Here's how the part is built. I have some questions about the finished solid (model axes, mm). Round coordinates to 2 decimals unless told otherwise and drop trailing zeros. Order: outer loops, then holes, each group sorted by start corner. A loop starts at its lowest first (then second) coordinate and runs counter-clockwise, first axis right, second up.
```python
from build123d import *

# Parameters (mm, degrees)
F0_R     = 31.75
F0_R_2   = 24.638
F1_DEPTH = 12.7
F2_R     = 3.175
F3_W     = 32.752518
F3_H     = 69.030817
F4_DEPTH = 15.875


with BuildPart() as f1:
    # F0 (on Front) → F1 (new body, symmetric)
    with BuildSketch(Plane.XZ):
        Circle(F0_R)
        Circle(F0_R_2, mode=Mode.SUBTRACT)
    extrude(amount=F1_DEPTH, both=True)

    # F2
    f2_edges = [f1.edges().sort_by_distance(p)[0] for p in [
        (-31.75, -12.7, 0),
        (-31.75, 12.7, 0),
    ]]
    fillet(f2_edges, radius=F2_R)

    # F3 (on Front) → F4 (cut, symmetric)
    with BuildSketch(Plane.XZ):
        with Locations((-16.376259, -0.200259)):
            Rectangle(F3_W, F3_H)
    extrude(amount=F4_DEPTH, both=True, mode=Mode.SUBTRACT)


solid = f1.part
```
1. If we mould it in two halves opening along Z, with no side actions, what happens to faces 1 (the cylindrical face through (24.632, 0.178, -0.542)), 2 (the cylindrical face through (31.742, -0.133, -0.698)), 3 (the flat face through (0, 0, 28))? For each: released by +Z, released by -Z, zero draft, split by the parting line, or undercut.
Evaluation:
face 1: undercut
face 2: split by the parting line
face 3: zero draft
2. I need wall thicknesses on probe 1 along Z at (x, y) = (16, 6); probe 2 along Z at (x, y) = (6.5, 7.5); probe 3 along X at (y, z) = (-11.5, 10). Which ranges of each line are inside material? Lowest first, please.
Evaluation:
probe 1: z = -27.42 to -18.74, 18.74 to 27.42
probe 2: z = -31.08 to -23.77, 23.77 to 31.08
probe 3: x = 22.52 to 29.41
3. If we section it at A-A, the plane z = 0: Write out the boundary of the cut face in (x, y) (3 decimals), and give its area (3 significant figures).
Evaluation:
outline: (24.638, -12.7) - (28.575, -12.7) arc R3.175 ccw to (31.75, -9.525) - (31.75, 9.525) arc R3.175 ccw to (28.575, 12.7) - (24.638, 12.7) - close
area: 176 mm2
4. If we section it at B-B, the plane y = -6: Write out the boundary of the cut face in (x, z), and give its area (3 significant figures).
Evaluation:
outline: (0, -31.75) arc R31.75 ccw to (0, 31.75) - (0, 24.64) arc R24.64 cw to (0, -24.64) - close
area: 630 mm2
5. I'm going to push flat-ended pins straight in: P1, Ø3, axis at x = 26, y = -1, coming from the -Z side; P2, Ø1, axis at x = 26, z = -17, coming from the -Y side; P3, Ø3, axis at y = -7.5, z = 11.5, coming from the +X side. Where does each tip first touch, or does it pass through?
Evaluation:
P1: stops at z = -20.19
P2: stops at y = -12
P3: stops at x = 30.13
